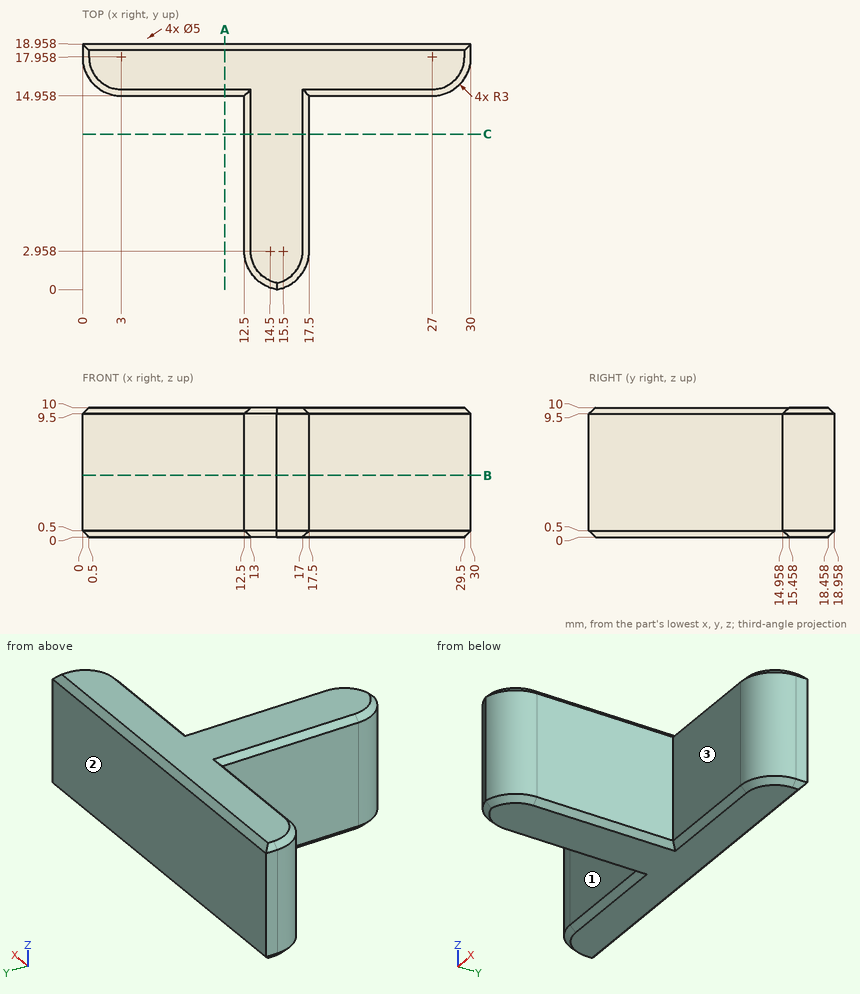
Here's the drawing with two shaded views (mm, measured from the low corner). I have some questions. A direction names the side the tool comes from. Give positions to 0.01 mm unless a question says otherwise; leave off trailing zeros. Order: outer loops, then holes, each group sorted by start corner. A loop starts at its lowest first (then second) coordinate and runs counter-clockwise, first axis right, second up. Notation, with made-up numbers: (-11.5, -33.5) -> (1.5, -33.5) arc R24 cw to (1.5, 3.5) -> close; hole circle Ø2 at (27.5, -34.75). An arc over 180 degrees is marked (long way). One line per item, written item: value. Start each with the question number.
1. Imagine slicing it at A-A, the plane x = 11. List the corners of the cut face in (y, z) for me.
2. Imagine slicing it at B-B, the plane z = 4.75. List the corners of the cut face in (x, y) for me, plus the area to 3 significant figures.
3. I need wall thicknesses on probe 1 along X at (y, z) = (10.5, 5.25); probe 2 along Y at (x, z) = (9, 8); probe 3 along Y at (x, z) = (28, 8.5). Which ranges of each line are inside material? Lowest first, please. Write a range as from..to.
4. Will these pins go through, and if not, where does the flat tip stop? pin 1 Ø2.5 at (y, z) = (7, 5.5) entering from +X; pin 2 Ø1.5 at (y, z) = (7.5, 8) entering from -X; pin 3 Ø1 at (x, z) = (26, 1.5) entering from -Y.
5. For the marked faces 1, 2 and 3, which set-ups out of +Z, -Z, +X, -X, +Y, -Y let a thin tool reach every point of the face, with its end or its side?
6. Imagine slicing it at C-C, the plane y = 12. List the corners of the cut face in (x, z) for me, plus the area to 3 significant figures.
Values follow:
1. outline: (14.96, 0.5) -> (15.46, 0) -> (18.46, 0) -> (18.96, 0.5) -> (18.96, 9.5) -> (18.46, 10) -> (15.46, 10) -> (14.96, 9.5) -> close
2. outline: (0, 17.96) arc R3 ccw to (3, 14.96) -> (12.5, 14.96) -> (12.5, 2.96) arc R3 ccw to (15, 0) arc R3 ccw to (17.5, 2.96) -> (17.5, 14.96) -> (27, 14.96) arc R3 ccw to (30, 17.96) -> (30, 18.96) -> (0, 18.96) -> close
2. area: 187 mm2
3. probe 1: x = 12.5..17.5
3. probe 2: y = 14.96..18.96
3. probe 3: y = 15.13..18.96
4. pin 1: stops at x = 17.5
4. pin 2: stops at x = 12.5
4. pin 3: stops at y = 14.96
5. face 1: +Z, -Z, -X, -Y
5. face 2: +Z, -Z, +X, -X, +Y
5. face 3: +Z, -Z, +X, -Y
6. outline: (12.5, 0.5) -> (13, 0) -> (17, 0) -> (17.5, 0.5) -> (17.5, 9.5) -> (17, 10) -> (13, 10) -> (12.5, 9.5) -> close
6. area: 49.5 mm2
